CAD build for the part. Positions are in the model's coordinates, mm. A direction names the side the tool comes from. Give positions to 0.01 mm unless a question says otherwise; leave off trailing zeros. Loops run counter-clockwise (first coordinate to the right, second up) from the corner with the lowest first, then second, coordinate; pieces in that order, holes last.
Item 1: Mould opens along Z. For faces 5 (the cylindrical face through (-176.07, 140.92, 27.8)), 6 (the cylindrical face through (-2.723, 22.255, 98.469)), 7 (the flat face through (-3, 65, -101.6)), 8 (the flat face through (2, 74, -95.25)) say: released by +Z, released by -Z, zero draft, split by the parting line, or undercut.
Item 2: Probe probe 1 along X at (y, z) = (143, -76.2); probe 2 along Z at (x, y) = (171, 139); probe 3 along X at (y, z) = (142, -25). List the from-to ranges inside material, lowest first.
Item 3: Which spindle directions (+Z, -Z, +X, -X, +Y, -Y) get a long thin tool onto all of the face, cutting with end or side? Do faces 1 (the flat face through (177.8, 0, 1)), 2 (the flat face through (171, 135.636, 1)), 3 (the flat face through (-172, 135.636, 1)), 4 (the cylindrical face through (166.25, 140.92, 25.17)). Say none if no direction does.
Item 4: Saw through at D-D on z = -16. Give the cut face in (x, y), plus the area to 3 significant figures.
Item 5: Saw through at B-B on x = -171.45. Give the cut face in (y, z).
Item 6: Saw through at C-C on x = 0. Give the cut face in (y, z) (3 decimals).
Item 7: Saw through at A-A on z = 76.2. Give the cut face in (x, y), plus the area to 3 significant figures.
Item 8: Drop flat-ended pins along their axis: P1, Ø1.5, axis at y = 65.5, z = -74.5, coming from the +X side; P2, Ø8, axis at x = 41, y = 123, coming from the +Z side; P3, Ø9.5, axis at x = -171.45, z = -76.2, coming from the +Y side. Give the stop position or say it passes through.
from build123d import *

# Parameters (mm, degrees)
BOSS_EXTRUDE1_DEPTH = 101.6
CUT_EXTRUDE1_DEPTH  = 95.25
CUT_EXTRUDE2_REACH  = 316.501
SKETCH5_R           = 123.825
SKETCH6_R           = 38.1
CUT_EXTRUDE3_DEPTH  = 311.436426664
SKETCH7_R           = 5.207
CUT_EXTRUDE4_DEPTH  = 83.566


with BuildPart() as part:
    # Sketch2 → Boss-Extrude1 (new, symmetric)
    with BuildSketch(Plane.XY):
        with BuildLine():
            Line((-190.5, 135.636), (-152.043772, 135.636))
            ThreePointArc((-152.043772, 135.636), (0, -6.35), (152.043772, 135.636))
            Line((152.043772, 135.636), (190.5, 135.636))
            Line((190.5, 135.636), (190.5, 146.05))
            Line((190.5, 146.05), (152.4, 146.05))
            Line((152.4, 146.05), (-152.4, 146.05))
            Line((-152.4, 146.05), (-190.5, 146.05))
            Line((-190.5, 146.05), (-190.5, 135.636))
        make_face()
        with BuildLine():
            Line((-84.242269675, 19.05), (-177.8, 19.05))
            Line((-177.8, 19.05), (-177.8, -19.05))
            Line((-177.8, -19.05), (177.8, -19.05))
            Line((177.8, -19.05), (177.8, 19.05))
            Line((177.8, 19.05), (84.242269675, 19.05))
            ThreePointArc((84.242269675, 19.05), (0, -6.35), (-84.242269675, 19.05))
        make_face()
    extrude(amount=BOSS_EXTRUDE1_DEPTH, both=True)

    # Sketch4 → Cut-Extrude1 (cut, symmetric)
    with BuildSketch(Plane.XY):
        with BuildLine():
            Line((-146.05, 146.05), (146.05, 146.05))
            ThreePointArc((146.05, 146.05), (0, 0), (-146.05, 146.05))
        make_face()
    extrude(amount=CUT_EXTRUDE1_DEPTH, both=True, mode=Mode.SUBTRACT)

    # Sketch5 → Cut-Extrude2 (cut, up to next)
    with BuildSketch(Plane.XY.offset(101.6), mode=Mode.PRIVATE) as cut_extrude2_sk1:
        with Locations((0, 146.05)):
            Circle(SKETCH5_R)
    cut_extrude2_tool1 = extrude(cut_extrude2_sk1.sketch, amount=-CUT_EXTRUDE2_REACH, mode=Mode.PRIVATE) & part.part
    add(cut_extrude2_tool1.solids().sort_by_distance((0, 146.05, 101.6))[0], mode=Mode.SUBTRACT)

    # Sketch6 → Cut-Extrude3 (cut, through all)
    with BuildSketch(Plane.XY.offset(-95.25)):
        with Locations((0, 146.05)):
            Circle(SKETCH6_R)
    extrude(amount=-CUT_EXTRUDE3_DEPTH, mode=Mode.SUBTRACT)

    # Sketch7 → Cut-Extrude4 (cut)
    with BuildSketch(Plane(origin=(0, 146.05, 0), x_dir=(1, 0, 0), z_dir=(0, 1, 0))):
        with Locations(Location((-171.45, 76.2, 0), (0, 0, 270))):
            Circle(SKETCH7_R)
        with Locations(Location((-171.45, 25.4, 0), (0, 0, 270))):
            Circle(SKETCH7_R)
        with Locations(Location((-171.45, -25.4, 0), (0, 0, 270))):
            Circle(SKETCH7_R)
        with Locations(Location((-171.45, -76.2, 0), (0, 0, 270))):
            Circle(SKETCH7_R)
        with Locations((171.45, -76.2)):
            Circle(SKETCH7_R)
        with Locations((171.45, -25.4)):
            Circle(SKETCH7_R)
        with Locations((171.45, 25.4)):
            Circle(SKETCH7_R)
        with Locations((171.45, 76.2)):
            Circle(SKETCH7_R)
    extrude(amount=-CUT_EXTRUDE4_DEPTH, mode=Mode.SUBTRACT)


solid = part.part
Results below:
1. face 5: undercut
1. face 6: zero draft
1. face 7: released by -Z
1. face 8: undercut
2. probe 1: x = -190.5 to -176.66, -166.24 to -146.02, 146.02 to 166.24, 176.66 to 190.5
2. probe 2: z = -101.6 to -81.39, -71.01 to -30.59, -20.21 to 20.21, 30.59 to 71.01, 81.39 to 101.6
2. probe 3: x = -190.5 to -176.64, -166.26 to -145.99, 145.99 to 166.26, 176.64 to 190.5
3. face 1: +Z, -Z, +X, -Y
3. face 2: +Z, -Z, +X
3. face 3: +Z, -Z, -X
3. face 4: +Y
4. outline: (-190.5, 135.64) - (-152.04, 135.64) arc R152.4 ccw to (-84.24, 19.05) - (-177.8, 19.05) - (-177.8, -19.05) - (177.8, -19.05) - (177.8, 19.05) - (84.24, 19.05) arc R152.4 ccw to (152.04, 135.64) - (190.5, 135.64) - (190.5, 146.05) - (146.05, 146.05) arc R146.05 cw to (-146.05, 146.05) - (-190.5, 146.05) - close
4. area: 14,400 mm2
5. outline: (-19.05, -101.6) - (19.05, -101.6) - (19.05, 101.6) - (-19.05, 101.6) - close; (135.64, -101.6) - (146.05, -101.6) - (146.05, -81.41) - (135.64, -81.41) - close; (135.64, -70.99) - (146.05, -70.99) - (146.05, -30.61) - (135.64, -30.61) - close; (135.64, -20.19) - (146.05, -20.19) - (146.05, 20.19) - (135.64, 20.19) - close; (135.64, 30.61) - (146.05, 30.61) - (146.05, 70.99) - (135.64, 70.99) - close; (135.64, 81.41) - (146.05, 81.41) - (146.05, 101.6) - (135.64, 101.6) - close
6. outline: (-19.05, -101.6) - (107.95, -101.6) - (107.95, -95.25) - (0, -95.25) - (0, 95.25) - (22.225, 95.25) - (22.225, 101.6) - (-19.05, 101.6) - close
7. outline: (-190.5, 135.64) - (-176.66, 135.64) - (-176.66, 146.05) - (-190.5, 146.05) - close; (-177.8, -19.05) - (177.8, -19.05) - (177.8, 19.05) - (84.24, 19.05) arc R152.4 ccw to (152.04, 135.64) - (166.24, 135.64) - (166.24, 146.05) - (146.05, 146.05) arc R146.05 cw to (-146.05, 146.05) - (-166.24, 146.05) - (-166.24, 135.64) - (-152.04, 135.64) arc R152.4 ccw to (-84.24, 19.05) - (-177.8, 19.05) - close; (176.66, 135.64) - (190.5, 135.64) - (190.5, 146.05) - (176.66, 146.05) - close
7. area: 14,200 mm2
8. P1: stops at x = 129.84
8. P2: stops at z = -95.25
8. P3: stops at y = 19.05
